Input: dimensioned drawing with shaded views. Units: mm. Origin: part minimum x, y, z. A direction names the side the tool comes from. Give positions to 0.01 mm unless a question says otherwise; leave off trailing zeros. Loops run counter-clockwise (first coordinate to the right, second up) from the corner with the lowest first, then second, coordinate; pieces in that order, holes last. Notation, with made-up numbers: (36, 38) -> (91, 38) arc R16 ccw to (91, 48) -> close; hole circle Ø3 at (-10.75, -10.75). An arc over 180 degrees is marked (long way). Answer as a JSON object with one key per item and string values.
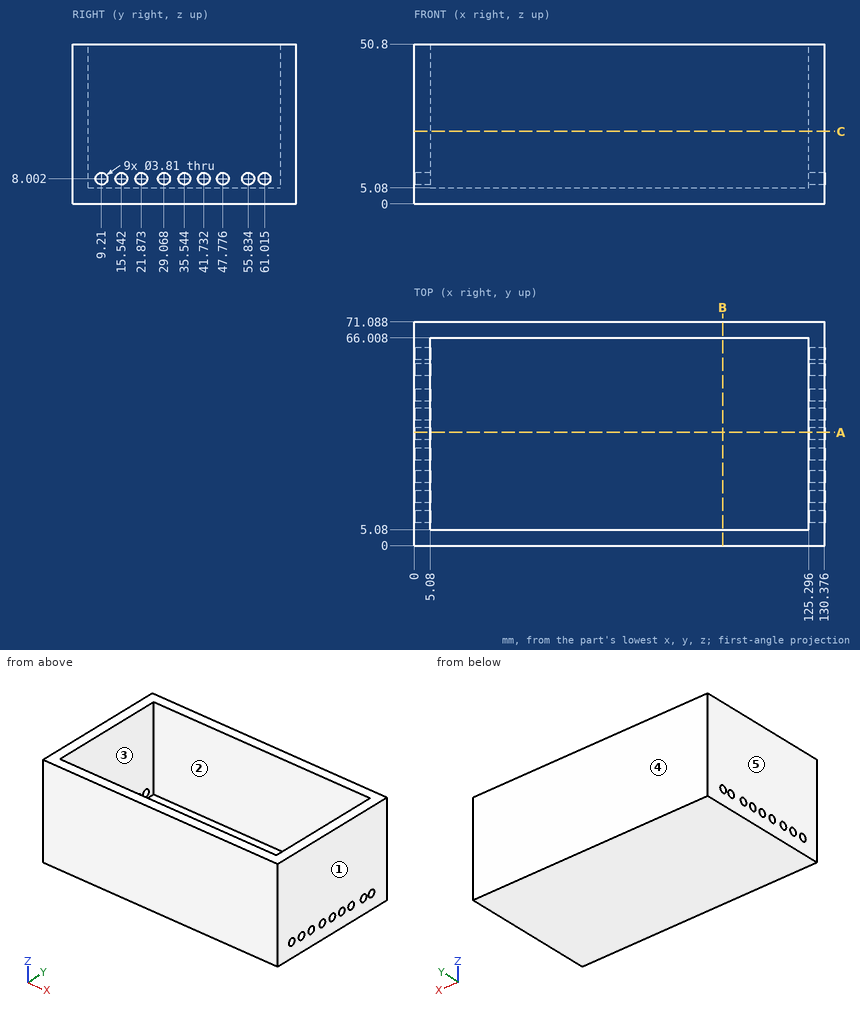
Q1. Section A-A, the plane y = 36. Return the cut outline in (x, z), then the cut area to 3 significant figures.
Evaluation:
{"outline": "(0, 0) -> (130.38, 0) -> (130.38, 6.15) -> (125.3, 6.15) -> (125.3, 5.08) -> (5.08, 5.08) -> (5.08, 6.15) -> (0, 6.15) -> close; (0, 9.85) -> (5.08, 9.85) -> (5.08, 50.8) -> (0, 50.8) -> close; (125.3, 9.85) -> (130.38, 9.85) -> (130.38, 50.8) -> (125.3, 50.8) -> close", "area": "1,090 mm2"}
Q2. Pin query (flat end, axial travel): pin 1 (3.5 mm diameter, centred on y = 21.87, z = 8, fed in from +X); pin 2 (6 mm diameter, centred on x = 45, y = 24.5, fed in from +Z). Return the tip coordinate at first contact, or that it passes through.
Evaluation:
{"pin 1": "passes through", "pin 2": "stops at z = 5.08"}
Q3. Draft query along X for the marked faces 3, 4 and 5. Return one class per face: +X half, -X half, draft (parallel to the pull), parting line (faces both ways), or undercut.
Evaluation:
{"face 3": "undercut", "face 4": "draft", "face 5": "-X half"}
Q4. Section C-C, the plane z = 23. Return the cut outline in (x, y).
Evaluation:
{"outline": "(0, 0) -> (130.38, 0) -> (130.38, 71.09) -> (0, 71.09) -> close; hole (5.08, 5.08) -> (125.3, 5.08) -> (125.3, 66.01) -> (5.08, 66.01) -> close"}
Q5. Ray query, line 1 along Y through (x, z) = (49, 40); line 2 along X through (y, z) = (12.5, 11); line 3 along Z through (x, y) = (86, 10). Return the intervals inside material, ascending.
Evaluation:
{"line 1": "y = 0 to 5.08, 66.01 to 71.09", "line 2": "x = 0 to 5.08, 125.3 to 130.38", "line 3": "z = 0 to 5.08"}
Q6. Access query for the marked faces 1 and 2. Directions: +Z, -Z, +X, -X, +Y, -Y. A direction counts if a zero-diameter tool reaches every point of the face in a straight line with its end or side. Return the directions, or none.
Evaluation:
{"face 1": "+Z, -Z, +X, +Y, -Y", "face 2": "+Z"}
Q7. Section B-B, the plane x = 98. Return the cut outline in (y, z).
Evaluation:
{"outline": "(0, 0) -> (71.09, 0) -> (71.09, 50.8) -> (66.01, 50.8) -> (66.01, 5.08) -> (5.08, 5.08) -> (5.08, 50.8) -> (0, 50.8) -> close"}
